For this review, use the dimensioned drawing (mm, ordinates from the lowest corner) and the shaded views. A direction names the side the tool comes from. Round coordinates to 2 decimals unless told otherwise and drop trailing zeros. Write each loop counter-clockwise with the first axis right and the second up, starting at its lowest first coordinate (ties: lowest second). Pieces come first, ordered by that corner, then holes. Notation, with made-up numbers: (17.5, 72.25) -> (36.5, 72.25) arc R12 ccw to (36.5, 89.25) -> close; hole circle Ø2 at (6.25, 18.25). An arc over 180 degrees is marked (long way). Write each question's results on one line, items separated by ' | '. Start each with the question number.
Item 1: To check wall thickness, follow line 1 along Y through (x, z) = (25.4, 37.45); line 2 along Z through (x, y) = (25.4, 0.8); line 3 along Y through (x, z) = (9, 34.5) (1 decimal). State the ranges of each line that lie inside material, in increasing order.
Item 2: Add section A-A (x = 25.4). State the section outline as (y, z) points (1 decimal).
Item 3: Clearance check with flat-ended pins moving along their axes: pin 1 (12 mm diameter, centred on x = 47.5, y = 13.5, fed in from -Z) (1 decimal); pin 2 (5 mm diameter, centred on x = 54.5, z = 22, fed in from +Y) (1 decimal); pin 3 (7.5 mm diameter, centred on x = 25.4, z = 17.46, fed in from -Y). State where each tip first meets the part, or that it passes through.
Item 4: Add section B-B (x = 135.5). State the section outline as (y, z) points (1 decimal).
Item 5: Add section C-C (z = 4.5). State the section outline as (x, y) points (1 decimal).
Item 6: Tool access review of the marked faces 1 and 2: name each direction out of +Z, -Z, +X, -X, +Y, -Y from which nothing blocks a thin tool from reaching the whole face with its end or side.
Item 7: Add section D-D (y = 6.5). State the section outline as (x, z) points (1 decimal).
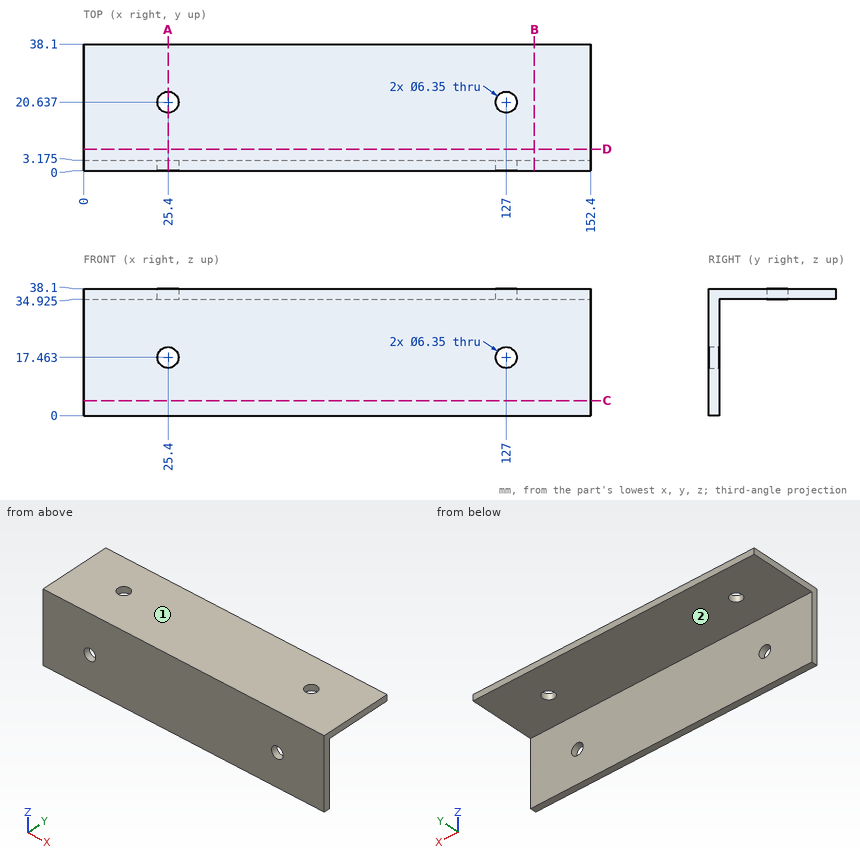
Responses:
1) line 1: y = 0 to 17.46, 23.81 to 38.1 | line 2: z = 0 to 14.29, 20.64 to 38.1 | line 3: y = 0 to 3.2
2) outline: (0, 0) -> (3.2, 0) -> (3.2, 14.3) -> (0, 14.3) -> close; (0, 20.6) -> (3.2, 20.6) -> (3.2, 34.9) -> (17.5, 34.9) -> (17.5, 38.1) -> (0, 38.1) -> close; (23.8, 34.9) -> (38.1, 34.9) -> (38.1, 38.1) -> (23.8, 38.1) -> close
3) pin 1: stops at z = 34.9 | pin 2: stops at y = 3.2 | pin 3: stops at y = 0
4) outline: (0, 0) -> (3.2, 0) -> (3.2, 34.9) -> (38.1, 34.9) -> (38.1, 38.1) -> (0, 38.1) -> close
5) outline: (0, 0) -> (152.4, 0) -> (152.4, 3.2) -> (0, 3.2) -> close
6) face 1: +Z, +X, -X, +Y, -Y | face 2: -Z, +X, -X, +Y
7) outline: (0, 34.9) -> (152.4, 34.9) -> (152.4, 38.1) -> (0, 38.1) -> close
